Verification items for the finished model (mm, model axes). A direction names the side the tool comes from. Round coordinates to 2 decimals unless told otherwise and drop trailing zeros. Write each loop counter-clockwise with the first axis right and the second up, starting at its lowest first coordinate (ties: lowest second). Pieces come first, ordered by that corner, then holes. Notation, with made-up numbers: (67.5, 88) -> (82.5, 88) arc R17 cw to (82.5, 114) -> close; hole circle Ø10 at (-20.75, 26.25). An arc over 180 degrees is marked (long way). Answer as a JSON object with one key per item and string values. Group by question number.
(1) Scan lines: L1, parallel to Y at x = 29, z = -0.8; L2, parallel to Y at x = 24, z = -4; L3, parallel to Z at x = 12.5, y = 6.25. Record each from-to range of solid material in increasing order. Write a range as from..to.
(2) Set-up check for faces 4 (the face through (28.594, 2.301, -12.715)), 5 (the face through (29, 0, -8)): record each of +Z, -Z, +X, -X, +Y, -Y from which the full face is reachable in a straight line by a thin tool's end or side.
(3) Sectioned sample at D-D on y = 8.5. Record the cut outline in (x, z), and give its area (3 significant figures).
(4) Draft check along X on faces 1 (the face through (29, 17, -7)), 2 (the face through (58, 8, -1)), 3 (the face through (32, 8.6, -14)). Enter one of: released by +X, released by -X, zero draft, split by the parting line, or undercut.
(5) Sectioned sample at A-A on y = 12. Record the cut outline in (x, z).
(6) Gauge pin test, flat end, axial feed: pin 1 Ø5 at (x, y) = (29, 8.5) entering from +Z. Record the tip position at first contact, or that the pin passes through.
(7) Sectioned sample at B-B on x = 53. Record the cut outline in (y, z), and give its area (3 significant figures).
(8) Sectioned sample at C-C on z = -7.75. Record the cut outline in (x, y), and give its area (3 significant figures).
Autodesk Inventor part; units mm, degrees
ref_plane "YZ Plane" through (0, 0, 0) normal (1, 0, 0) x (0, 1, 0)
ref_plane "XZ Plane" through (0, 0, 0) normal (0, 1, 0) x (-1, 0, 0)
ref_plane "XY Plane" through (0, 0, 0) normal (0, 0, 1) x (1, 0, 0)
sketch "Sketch2" plane through (0, 0, 0) normal (1, 0, 0) x (0, 1, 0)
  line L0 (0, 0) -> (17, 0)
  line L1 (17, 0) -> (17, -15)
  line L2 (17, -15) -> (0, -15)
  line L3 (0, -15) -> (0, 0)
  dimension "d4" = 17
  dimension "d5" = 15
extrude "Extrusion2" add sketch "Sketch2" along normal blind 58
sketch "Sketch3" plane through (58, 0, 0) normal (1, 0, 0) x (0, 0, -1)
  line L0 (0, 17) -> (0, 0)
  line L1 (0, 0) -> (15, 0)
  line L2 (15, 0) -> (15, 17)
  line L3 (2, 2) -> (13, 2)
  line L4 (13, 2) -> (13, 15)
  line L5 (13, 15) -> (2, 15)
  line L6 (2, 15) -> (2, 2)
  line L7 (2, 2) -> (13, 15) construction
  line L8 (13, 2) -> (2, 15) construction
  point P0 (7.5, 8.5)
  dimension "d9" = 11
  dimension "d10" = 13
extrude "Extrusion3" cut sketch "Sketch3" against normal through all
sketch "Sketch5" plane through (0, 0, -15) normal (0, 0, -1) x (-1, 0, 0)
  line L0 (0, 0) -> (-58, 0)
  line L1 (-58, 0) -> (0, 17)
  line L2 (-58, 0) -> (-58, 17)
  line L3 (0, 0) -> (-58, 17)
  circle A0 centre (-29, 8.5) radius 3
  dimension "d13" = 6
extrude "Extrusion4" cut sketch "Sketch5" against normal through all contours A0 L1 L3 | L3 L1 A0 | A0 L3 L1 | L3 A0 L1
fillet "Fillet1" radius 1 4 edges at (29, 2, -13) (29, 2, -2) (29, 15, -2) (29, 15, -13)
properties part number "caja perfil"
Computed values:
{
 "1": {"L1": "0..5.5, 11.5..17", "L2": "0..2, 15..17", "L3": "-15..-13, -2..0"},
 "2": {"face 4": "+X, -X", "face 5": "+Z, -Z, +X, -X, -Y"},
 "3": {"outline": "(0, -15) -> (26, -15) -> (26, -13) -> (0, -13) -> close; (0, -2) -> (26, -2) -> (26, 0) -> (0, 0) -> close; (32, -15) -> (58, -15) -> (58, -13) -> (32, -13) -> close; (32, -2) -> (58, -2) -> (58, 0) -> (32, 0) -> close", "area": "208 mm2"},
 "4": {"face 1": "zero draft", "face 2": "released by +X", "face 3": "undercut"},
 "5": {"outline": "(0, -15) -> (58, -15) -> (58, -13) -> (0, -13) -> close; (0, -2) -> (58, -2) -> (58, 0) -> (0, 0) -> close"},
 "6": {"pin 1": "through"},
 "7": {"outline": "(0, -15) -> (17, -15) -> (17, 0) -> (0, 0) -> close; hole (2, -12) arc R1 ccw to (3, -13) -> (14, -13) arc R1 ccw to (15, -12) -> (15, -3) arc R1 ccw to (14, -2) -> (3, -2) arc R1 ccw to (2, -3) -> close", "area": "113 mm2"},
 "8": {"outline": "(0, 0) -> (58, 0) -> (58, 2) -> (0, 2) -> close; (0, 15) -> (58, 15) -> (58, 17) -> (0, 17) -> close", "area": "232 mm2"}
}
